Geometry: final body of the model. Coordinates: model frame, mm. Round coordinates to 2 decimals unless told otherwise and drop trailing zeros. Loops run counter-clockwise (first coordinate to the right, second up) from the corner with the lowest first, then second, coordinate; pieces in that order, holes last. Notation, with made-up numbers: (44.25, 75.5) - (77.25, 75.5) arc R32 ccw to (77.25, 103.5) - close; hole circle Ø1 at (26, -5). An arc over 180 degrees is marked (long way). Write item = value, one per line. Start each with the question number.
Item 1: Section D-D (y = 1.25). Return loops of the section in (x, z).
Item 2: Line query: line 1 (Y direction, x = 37, z = 1.1); line 2 (X direction, y = 2, z = 0.65); line 3 (Y direction, x = 3, z = 1.8). Output: solid intervals per line, ascending. Write a range as from..to.
Item 3: First-contact query: pin 1 (1 mm diameter, centred on y = 6, z = 1.5, fed in from +X); pin 2 (0.8 mm diameter, centred on x = -5, z = 1, fed in from -Y). Flat tips, straight axial feed; report the tip coordinate or a pass-through.
Item 4: Section B-B (z = 1.25). Return loops of the section in (x, y), plus the area to 3 significant figures.
Item 5: Section A-A (x = 6.5). Return loops of the section in (y, z).
Item 6: Section C-C (x = 34). Return loops of the section in (y, z).
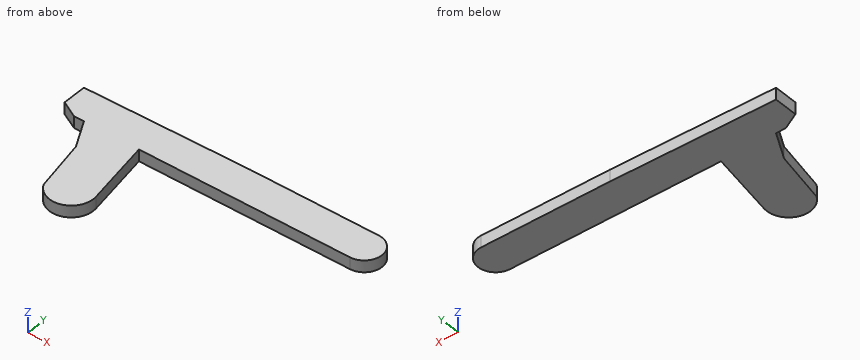
from build123d import *

# Parameters (mm, degrees)
F1_DEPTH = 2


with BuildPart() as f1:
    # F0 (on Top) → F1 (new body)
    with BuildSketch(Plane.XY):
        with BuildLine():
            ThreePointArc((41.035574, 8.848914), (44.035574, 11.848914), (41.035574, 14.848914))
            Line((41.035574, 14.848914), (19.065223, 14.848914))
            Line((19.065223, 14.848914), (-8.964426, 14.368003))
            Line((-8.964426, 14.368003), (-8.964426, 10.348275))
            Line((-8.964426, 10.348275), (-6.120325, 8.848914))
            Line((-6.120325, 8.848914), (-4.4251, 8.848914))
            Line((-4.4251, 8.848914), (-1.831835, 4.020077))
            Line((-1.831835, 4.020077), (0, -4.946886))
            ThreePointArc((0, -4.946886), (4.5255, -6.684783), (6.973939, -2.500816))
            Line((6.973939, -2.500816), (4.972675, 8.848914))
            Line((4.972675, 8.848914), (41.035574, 8.848914))
        make_face()
    extrude(amount=F1_DEPTH)


solid = f1.part
Taken from the geometry:
q1.outline = (-1.27, 0) - (6.31, 0) - (6.31, 2) - (-1.27, 2) - close
q2.line_1 = 8.85..14.85
q2.line_2 = -1.42..6.18
q2.line_3 = -6.88..14.57
q3.pin_1 = 5.56
q3.pin_2 = 8.85
q4.outline = (-8.96, 10.35) - (-6.12, 8.85) - (-4.43, 8.85) - (-1.83, 4.02) - (0, -4.95) arc R3.74 ccw to (6.97, -2.5) - (4.97, 8.85) - (41.04, 8.85) arc R3 ccw to (41.04, 14.85) - (19.07, 14.85) - (-8.96, 14.37) - close
q4.area = 422 mm^2
q5.outline = (-5.07, 0) - (0.19, 0) - (0.19, 2) - (-5.07, 2) - close; (8.85, 0) - (14.63, 0) - (14.63, 2) - (8.85, 2) - close
q6.outline = (8.85, 0) - (14.85, 0) - (14.85, 2) - (8.85, 2) - close
